Geometry: final body of the model. Coordinates: model frame, mm. Round coordinates to 2 decimals unless told otherwise and drop trailing zeros. Loops run counter-clockwise (first coordinate to the right, second up) from the corner with the lowest first, then second, coordinate; pieces in that order, holes last. Notation, with made-up numbers: (31.25, 71) - (53.25, 71) arc R32 ccw to (53.25, 103) - close; hole circle Ø9 at (-18.75, 31.25). An arc over 180 degrees is marked (long way). Return JSON: item names as keys, results as strings. Group by question number.
1. Material intervals for probe 1 along X at (y, z) = (26, 1.95); probe 2 along Y at (x, z) = (-12.5, 2.6); probe 3 along Y at (x, z) = (9, 3.75), sorted ascending.
2. Section B-B on z = 2.7. Return loops of the section in (x, y).
3. Draft query along X for faces 1 (the face through (-12.695, 26.487, 2.535)), 2 (the face through (-2.38, -10.74, 2.46)), 3 (the face through (25, 24, 3)), 4 (the face through (0.55, -24.994, 2.535)). Return one class per face: +X half, -X half, draft (parallel to the pull), parting line (faces both ways), or undercut.
4. Section A-A on x = 0. Return loops of the section in (y, z), and give its area (3 significant figures).
5. Section C-C on y = 2. Return loops of the section in (x, z), and give its area (3 significant figures).
6. First-contact query: pin 1 Ø2.5 at (x, y) = (-12.5, 25) entering from +Z; pin 2 Ø1 at (x, z) = (12, 2.5) entering from -Y. Flat tips, straight axial feed; report the tip coordinate or a pass-through.
7. Section D-D on x = -15.5. Return loops of the section in (y, z).
from build123d import *

# Parameters (mm, degrees)
ESQUISSE1_W             = 94
ESQUISSE1_H             = 93.807810261
ESQUISSE1_R             = 11
BOSS_EXTRU_1_DEPTH      = 5
ESQUISSE2_R             = 1.5
ENL_V_MAT_EXTRU_1_DEPTH = 67.655832453


with BuildPart() as part:
    # Esquisse1 → Boss.-Extru.1 (new body)
    with BuildSketch(Plane.XY):
        with Locations((0, 0.096094869)):
            Rectangle(ESQUISSE1_W, ESQUISSE1_H)
        Circle(ESQUISSE1_R, mode=Mode.SUBTRACT)
    extrude(amount=BOSS_EXTRU_1_DEPTH)

    # Esquisse2 → Enlèv. mat.-Extru.1 (cut, through all)
    with BuildSketch(Plane.XY.offset(5)):
        with BuildLine():
            Line((25, 47), (25, 0))
            ThreePointArc((25, 0), (0, -25), (-25, 0))
            Line((-25, 0), (-25, 47))
            Line((-25, 47), (-47, 47))
            Line((-47, 47), (-47, -46.807810261))
            Line((-47, -46.807810261), (47, -46.807810261))
            Line((47, -46.807810261), (47, 47))
            Line((47, 47), (25, 47))
        make_face()
        with Locations((-12.5, 25)):
            Circle(ESQUISSE2_R)
        with Locations((12.5, 25)):
            Circle(ESQUISSE2_R)
    extrude(amount=-ENL_V_MAT_EXTRU_1_DEPTH, mode=Mode.SUBTRACT)


solid = part.part
Taken from the geometry:
{
 "1": {"probe 1": "-25 to -13.62, -11.38 to 11.38, 13.62 to 25", "probe 2": "-21.65 to 23.5, 26.5 to 47", "probe 3": "-23.32 to -6.32, 6.32 to 47"},
 "2": {"outline": "(-25, 0) arc R25 ccw to (25, 0) - (25, 47) - (-25, 47) - close; hole circle Ø3 at (-12.5, 25); hole circle Ø22 at (0, 0); hole circle Ø3 at (12.5, 25)"},
 "3": {"face 1": "undercut", "face 2": "undercut", "face 3": "+X half", "face 4": "parting line"},
 "4": {"outline": "(-25, 0) - (-11, 0) - (-11, 5) - (-25, 5) - close; (11, 0) - (47, 0) - (47, 5) - (11, 5) - close", "area": "250 mm2"},
 "5": {"outline": "(-25, 0) - (-10.82, 0) - (-10.82, 5) - (-25, 5) - close; (10.82, 0) - (25, 0) - (25, 5) - (10.82, 5) - close", "area": "142 mm2"},
 "6": {"pin 1": "through", "pin 2": "y = -22.2"},
 "7": {"outline": "(-19.62, 0) - (47, 0) - (47, 5) - (-19.62, 5) - close"}
}
